Source: CAD feature listing. Evaluate the final solid. Frame: model axes, mm. Coordinates: 2 decimals unless noted, no trailing zeros. Order: outer loops, then holes, each group sorted by start corner. A loop starts at its lowest first (then second) coordinate and runs counter-clockwise, first axis right, second up. Notation, with made-up numbers: (72, -10) -> (126, -10) arc R22 ccw to (126, 9) -> close; hole circle Ø4 at (53, 33.5). An arc over 180 degrees is marked (long way). Write each question's results on one line, items separated by ' | '. Start each with the question number.
Autodesk Inventor part; units mm, degrees
ref_plane "YZ Plane" through (0, 0, 0) normal (1, 0, 0) x (0, 1, 0)
ref_plane "XZ Plane" through (0, 0, 0) normal (0, 1, 0) x (-1, 0, 0)
ref_plane "XY Plane" through (0, 0, 0) normal (0, 0, 1) x (1, 0, 0)
ref_plane "Work Plane1" through (-337.8481, -441.0413, 0) normal (0, 0, 1) x (1, 0, 0)
sketch "Sketch1" plane through (-337.8481, -441.0413, 0) normal (0, 0, 1) x (1, 0, 0)
  line L0 (-84.5, -47.3468) -> (-42.5, -47.3468)
  line L1 (-42.5, -47.3468) -> (-42.5, -5.3468)
  line L2 (-42.5, -5.3468) -> (-84.5, -5.3468)
  line L3 (-84.5, -5.3468) -> (-84.5, -47.3468)
  line L4 (-84.5, -47.3468) -> (-42.5, -5.3468) construction
  line L5 (-42.5, -47.3468) -> (-84.5, -5.3468) construction
  point P0 (337.8481, 441.0413)
  point P1 (-63.5, -26.3468)
  dimension "d0" = 42
  dimension "d1" = 42
extrude "Extrusion1" add sketch "Sketch1" against normal blind 50.8
sketch "Sketch2" plane through (-337.8481, -441.0413, -50.8) normal (0, 0, -1) x (-1, 0, 0)
  line L0 (42.5, -47.3468) -> (84.5, -47.3468)
  line L1 (84.5, -47.3468) -> (84.5, -5.3468)
  line L2 (84.5, -5.3468) -> (42.5, -5.3468)
  line L3 (42.5, -5.3468) -> (42.5, -47.3468)
  circle A0 centre (63.5, -26.3468) radius 6.35
  point P0 (-337.8481, 441.0413)
  dimension "d4" = 12.7
extrude "Extrusion2" add sketch "Sketch2" along normal blind 622.3 contours A0
sketch "Sketch3" plane through (-337.8481, -441.0413, -50.8) normal (0, 0, -1) x (-1, 0, 0)
  circle A0 centre (63.5, -26.3468) radius 6.35
  line L0 (42.5, -47.3468) -> (84.5, -47.3468)
  line L1 (84.5, -47.3468) -> (84.5, -5.3468)
  line L2 (84.5, -5.3468) -> (42.5, -5.3468)
  line L3 (42.5, -5.3468) -> (42.5, -47.3468)
  circle A1 centre (63.5, -26.3468) radius 19.05
  point P0 (-337.8481, 441.0413)
  dimension "d7" = 38.1
extrude "Extrusion3" add sketch "Sketch3" along normal blind 38.1 contours A1
sketch "Sketch4" plane through (-337.8481, -441.0413, -50.8) normal (0, 0, -1) x (-1, 0, 0)
  circle A0 centre (63.5, -26.3468) radius 19.05
  line L0 (42.5, -47.3468) -> (84.5, -47.3468)
  line L1 (84.5, -47.3468) -> (84.5, -5.3468)
  line L2 (84.5, -5.3468) -> (42.5, -5.3468)
  line L3 (42.5, -5.3468) -> (42.5, -47.3468)
  circle A1 centre (63.5, -26.3468) radius 6.35
  point P0 (-337.8481, 441.0413)
extrude "Extrusion4" cut sketch "Sketch4" along normal mid plane 5.08 contours A0 | L3 L2 L1 L0
properties part number "MotorandLeadscrew"
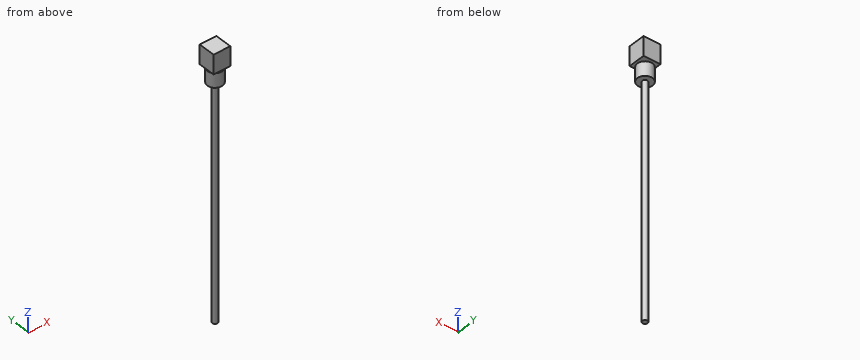
(1) First-contact query: P1, Ø12, axis at x = -399.5, z = -286, coming from the +Y side; P2, Ø8, axis at y = -475.5, z = -416.5, coming from the +X side; P3, Ø6, axis at y = -478, z = -131.5, coming from the +X side; P4, Ø6, axis at x = -407, z = -415, coming from the +Y side. Flat tips, straight axial feed; report the tip coordinate or a pass-through.
(2) Section A-A on x = -400.5. Return the cut outline in (y, z) (3 decimals).
(3) Line query: L1, parallel to Z at x = -396.5, y = -483; L2, parallel to Z at x = -420, y = -451.5; L3, parallel to X at y = -468, z = -574.5. Output: solid intervals per line, ascending.
(4) Section B-B on z = -507. Return the cut outline in (x, y).
Results list:
1) P1: stops at y = -461.04 | P2: stops at x = -396.51 | P3: passes through | P4: stops at y = -461.62
2) outline: (-488.388, -48.26) -> (-473.681, -48.26) -> (-473.681, -53.34) -> (-486.419, -53.34) -> (-486.419, -88.9) -> (-473.681, -88.9) -> (-473.681, -673.1) -> (-461.095, -673.1) -> (-461.095, -88.9) -> (-448.357, -88.9) -> (-448.357, -53.34) -> (-461.095, -53.34) -> (-461.095, -48.26) -> (-446.388, -48.26) -> (-446.388, 0) -> (-488.388, 0) -> close
3) L1: z = -88.9 to -53.34, -48.26 to 0 | L2: z = -48.26 to 0 | L3: x = -407.67 to -395.03
4) outline: circle Ø12.7 at (-401.35, -467.39)
